Autodesk Inventor part; units mm, degrees
ref_plane "YZ Plane" through (0, 0, 0) normal (1, 0, 0) x (0, 1, 0)
ref_plane "XZ Plane" through (0, 0, 0) normal (0, 1, 0) x (-1, 0, 0)
ref_plane "XY Plane" through (0, 0, 0) normal (0, 0, 1) x (1, 0, 0)
sketch "Sketch10" plane through (0, 0, 0) normal (0, 1, 0) x (-1, 0, 0)
  circle A0 centre (0, 0) radius 3.175
  circle A1 centre (0, 0) radius 5.715
  line L0 (0, 3.175) -> (0, 5.207)
  line L1 (0, 5.207) -> (2.3555, 5.207)
  line L2 (-2.3555, 5.207) -> (0, 5.207)
  dimension "d61" = 6.35
  dimension "d62" = 11.43
  dimension "d63" = 2.032
extrude "Extrusion7" add sketch "Sketch10" along normal blind 25.4 contours A1 L2 L1 picked at (-1.045, 4.4973)
sketch "Sketch12" plane through (-2.3555, 0, 5.207) normal (0, 0, 1) x (1, 0, 0)
  line L0 (2.3555, 0) -> (2.3555, 4.2418)
  line L1 (2.3555, 4.2418) -> (2.3555, 8.4836)
  line L2 (8.0705, 25.4) -> (-3.3595, 25.4)
  line L3 (2.3555, 25.4) -> (2.3555, 21.1582)
  line L4 (2.3555, 21.1582) -> (2.3555, 16.9164)
  point P0 (4.711, 25.4)
  point P1 (0, 25.4)
  dimension "d66" = 4.2418
  dimension "d67" = 4.2418
  dimension "d68" = 4.2418
  dimension "d69" = 4.2418
hole "Hole5" at (0, 21.1582, 5.207) at (0, 16.9164, 5.207) at (0, 8.4836, 5.207) at (0, 4.2418, 5.207) direction (0, 0, -1) diameter 1.567 depth 6.2992
properties part number "rotaryconnector"
Check sheet for the modelled part. Datum: model origin and axes. Units: mm. A direction names the side the tool comes from. Give positions to 0.01 mm unless a question says otherwise; leave off trailing zeros. Order: outer loops, then holes, each group sorted by start corner. A loop starts at its lowest first (then second) coordinate and runs counter-clockwise, first axis right, second up. Notation, with made-up numbers: (-12, -36) -> (23, -36) arc R20 cw to (23, -2) -> close; hole circle Ø1 at (-1.75, -25.75). An arc over 180 degrees is marked (long way). Use CSV: the item, a comma, the result in double quotes. Start each with the question number.
1) Sectioned sample at C-C, the plane z = 4.25. Record the boundary of the cut face in (x, y), plus the area to 3 significant figures.
2) Sectioned sample at B-B, the plane z = 0. Record the boundary of the cut face in (x, y) (3 decimals), plus the area to 3 significant figures.
3) Mould release check, pull along Z, two halves, no side actions. Record for faces 1 (the face through (-0.034, 9.266, 4.127)), 2 (the face through (0.41, 12.52, -3.15)), 3 (the face through (-0.22, 12.52, -5.71)), 4 (the face through (0, 13, 5.207)): released by +Z, released by -Z, zero draft, split by the parting line, or undercut.
4) Sectioned sample at A-A, the plane x = 0. Record the boundary of the cut face in (y, z) (3 decimals), plus the area to 3 significant figures.
5) Go/stop test with flat-tipped pins: P1, Ø2, axis at x = -3.5, y = 3, coming from the -Z side; P2, Ø1, axis at x = 1, y = 17.5, coming from the -Z side; P3, Ø1, axis at x = 2.5, y = 4.5, coming from the -Z side. Record where each tip stops, or that it passes through.
6) Set-up check for faces 5 (the face through (-2.5, 25.4, 2.2)), 6 (the face through (-0.24, 16.17, 4.13)): record each of +Z, -Z, +X, -X, +Y, -Y from which the full face is reachable in a straight line by a thin tool's end or side.
7) Material ranges on line 1 (Y direction, x = 0, z = 4.6); line 2 (X direction, y = 12, z = -1.5); line 3 (X direction, y = 1.25, z = 2), recorded low to high. Write a range as from..to.
Recorded:
1,outline,"(-3.82, 0) -> (3.82, 0) -> (3.82, 25.4) -> (-3.82, 25.4) -> close; hole circle Ø1.57 at (0, 4.24); hole circle Ø1.57 at (0, 8.48); hole circle Ø1.57 at (0, 16.92); hole circle Ø1.57 at (0, 21.16)"
1,area,"186 mm2"
2,outline,"(-5.715, 0) -> (-3.175, 0) -> (-3.175, 25.4) -> (-5.715, 25.4) -> close; (3.175, 0) -> (5.715, 0) -> (5.715, 25.4) -> (3.175, 25.4) -> close"
2,area,"129 mm2"
3,face 1,"zero draft"
3,face 2,"undercut"
3,face 3,"split by the parting line"
3,face 4,"released by +Z"
4,outline,"(0, -5.715) -> (25.4, -5.715) -> (25.4, -3.175) -> (0, -3.175) -> close; (0, 3.175) -> (3.458, 3.175) -> (3.458, 5.207) -> (0, 5.207) -> close; (5.025, 3.175) -> (7.7, 3.175) -> (7.7, 5.207) -> (5.025, 5.207) -> close; (9.267, 3.175) -> (16.133, 3.175) -> (16.133, 5.207) -> (9.267, 5.207) -> close; (17.7, 3.175) -> (20.375, 3.175) -> (20.375, 5.207) -> (17.7, 5.207) -> close; (21.942, 3.175) -> (25.4, 3.175) -> (25.4, 5.207) -> (21.942, 5.207) -> close"
4,area,"103 mm2"
5,P1,"z = -5.14"
5,P2,"z = -5.69"
5,P3,"z = -5.35"
6,face 5,"+Z, -Z, +X, -X, +Y"
6,face 6,"+Z"
7,line 1,"0..3.46, 5.03..7.7, 9.27..16.13, 17.7..20.37, 21.94..25.4"
7,line 2,"-5.51..-2.8, 2.8..5.51"
7,line 3,"-5.35..-2.47, 2.47..5.35"
